Check sheet for the modelled part. Datum: model origin and axes. Units: mm. A direction names the side the tool comes from. Give positions to 0.01 mm unless a question says otherwise; leave off trailing zeros. Use CSV: the item, a comma, the result in double quotes.
from build123d import *

# Parameters (mm, degrees)
SKETCH_1_W             = 23.5
SKETCH_1_H             = 12
EXTRUDE_1_DEPTH        = 650.5
HOLE_WIZARD_M6_1_D     = 5
HOLE_WIZARD_M6_1_DEPTH = 19
HOLE_WIZARD_M6_1_TIP   = 1.502151548
HOLE_WIZARD_M4_1_D     = 3.3
HOLE_WIZARD_M4_1_DEPTH = 15.5
HOLE_WIZARD_M4_1_TIP   = 0.991420021
HOLE_WIZARD_M6_2_D     = 5
HOLE_WIZARD_M6_2_DEPTH = 17
HOLE_WIZARD_M6_2_TIP   = 1.502151548
HOLE_WIZARD_M4_2_D     = 3.3
HOLE_WIZARD_M4_2_DEPTH = 11.5
HOLE_WIZARD_M4_2_TIP   = 0.991420021


with BuildPart() as part:
    # 草图1 → 凸台-拉伸1 (new, symmetric)
    with BuildSketch(Plane(origin=(0, 0, 0), x_dir=(0, 0, -1), z_dir=(1, 0, 0))):
        Polygon((-15, 15), (-11.5, 15), (-11.5, 13.5), (-11, 13.5), (-11, 12), (-9.5, 12), (-9.5, 15), (-8, 15), (-8, 12.5), (-5, 12.5), (-5, 15), (5, 15), (5, 12.5), (8, 12.5), (8, 15), (9.5, 15), (9.5, 12), (11, 12), (11, 13.5), (11.5, 13.5), (11.5, 15), (15, 15), (15, 8), (12.5, 8), (12.5, 5), (15, 5), (15, -5), (12.5, -5), (12.5, -8), (15, -8), (15, -15), (11.5, -15), (11.5, -13.5), (11, -13.5), (11, -12), (9.5, -12), (9.5, -15), (8, -15), (8, -12.5), (5, -12.5), (5, -15), (-5, -15), (-5, -12.5), (-8, -12.5), (-8, -15), (-9.5, -15), (-9.5, -12), (-11, -12), (-11, -13.5), (-11.5, -13.5), (-11.5, -15), (-15, -15), align=None)
        with BuildLine():
            Line((12, -10.5), (12, -8.5))
            ThreePointArc((12, -8.5), (11.853553391, -8.146446609), (11.5, -8))
            Line((11.5, -8), (-11.5, -8))
            ThreePointArc((-11.5, -8), (-11.853553391, -8.146446609), (-12, -8.5))
            Line((-12, -8.5), (-12, -10.5))
            ThreePointArc((-12, -10.5), (-11.853553391, -10.853553391), (-11.5, -11))
            Line((-11.5, -11), (11.5, -11))
            ThreePointArc((11.5, -11), (11.853553391, -10.853553391), (12, -10.5))
        make_face(mode=Mode.SUBTRACT)
        with BuildLine():
            Line((-11.5, 11), (11.5, 11))
            ThreePointArc((11.5, 11), (11.853553391, 10.853553391), (12, 10.5))
            Line((12, 10.5), (12, 8.5))
            ThreePointArc((12, 8.5), (11.853553391, 8.146446609), (11.5, 8))
            Line((11.5, 8), (-11.5, 8))
            ThreePointArc((-11.5, 8), (-11.853553391, 8.146446609), (-12, 8.5))
            Line((-12, 8.5), (-12, 10.5))
            ThreePointArc((-12, 10.5), (-11.853553391, 10.853553391), (-11.5, 11))
        make_face(mode=Mode.SUBTRACT)
        Rectangle(SKETCH_1_W, SKETCH_1_H, mode=Mode.SUBTRACT)
    extrude(amount=EXTRUDE_1_DEPTH, both=True)

    # M6 螺纹孔1
    with Locations(Plane(origin=(0, 0, -15), x_dir=(-1, 0, 0), z_dir=(0, 0, -1))):
        with Locations((-630.5, 0), (-615.5, 0), (342.5, 0), (327.5, 0), (427.5, 0), (412.5, 0), (630.5, 0), (615.5, 0)):
            Hole(HOLE_WIZARD_M6_1_D / 2, depth=HOLE_WIZARD_M6_1_DEPTH)
            with Locations((0, 0, -(HOLE_WIZARD_M6_1_DEPTH + HOLE_WIZARD_M6_1_TIP / 2))):  # 118° drill point
                Cone(0, HOLE_WIZARD_M6_1_D / 2, HOLE_WIZARD_M6_1_TIP, mode=Mode.SUBTRACT)

    # M4 螺纹孔1
    with Locations(Plane.XY.offset(15)):
        with Locations((-460, 0), (-230, 0), (0, 0), (230, 0), (460, 0)):
            Hole(HOLE_WIZARD_M4_1_D / 2, depth=HOLE_WIZARD_M4_1_DEPTH)
            with Locations((0, 0, -(HOLE_WIZARD_M4_1_DEPTH + HOLE_WIZARD_M4_1_TIP / 2))):  # 118° drill point
                Cone(0, HOLE_WIZARD_M4_1_D / 2, HOLE_WIZARD_M4_1_TIP, mode=Mode.SUBTRACT)

    # M6 螺纹孔2
    with Locations(Plane(origin=(0, -15, 0), x_dir=(-1, 0, 0), z_dir=(0, -1, 0))):
        with Locations((310.5, 0), (285.5, 0), (-285.5, 0), (-310.5, 0), (590.5, 0), (470.5, 0)):
            Hole(HOLE_WIZARD_M6_2_D / 2, depth=HOLE_WIZARD_M6_2_DEPTH)
            with Locations((0, 0, -(HOLE_WIZARD_M6_2_DEPTH + HOLE_WIZARD_M6_2_TIP / 2))):  # 118° drill point
                Cone(0, HOLE_WIZARD_M6_2_D / 2, HOLE_WIZARD_M6_2_TIP, mode=Mode.SUBTRACT)

    # M4 螺纹孔2
    with Locations(Plane(origin=(0, -15, 0), x_dir=(-1, 0, 0), z_dir=(0, -1, 0))):
        with Locations((642.5, 0), (615.5, 0)):
            Hole(HOLE_WIZARD_M4_2_D / 2, depth=HOLE_WIZARD_M4_2_DEPTH)
            with Locations((0, 0, -(HOLE_WIZARD_M4_2_DEPTH + HOLE_WIZARD_M4_2_TIP / 2))):  # 118° drill point
                Cone(0, HOLE_WIZARD_M4_2_D / 2, HOLE_WIZARD_M4_2_TIP, mode=Mode.SUBTRACT)


solid = part.part
1. Scan lines: line 1 along Y through (x, z) = (188, 7); line 2 along Y through (x, z) = (225.5, -3); line 3 along Z through (x, y) = (-497, -13.25). Record each from-to range of solid material in increasing order.
Completed:
line 1,"y = -12.5 to -11, -8 to -6, 6 to 8, 11 to 12.5"
line 2,"y = -15 to -11, -8 to -6, 6 to 8, 11 to 15"
line 3,"z = -15 to -11, -9.5 to -8, -5 to 5, 8 to 9.5, 11 to 15"
2. Go/stop test with flat-tipped pins: pin 1 Ø2 at (x, z) = (-615.5, 0) entering from -Y; pin 2 Ø5 at (y, z) = (1.5, 6.5) entering from +X. Record where each tip stops, or that it passes through.
Completed:
pin 1,"stops at y = 6"
pin 2,"passes through"
3. Set-up check for faces 4 (the face through (9, -6, 0)), 5 (the face through (-650.5, 7, 0)): record each of +Z, -Z, +X, -X, +Y, -Y from which the full face is reachable in a straight line by a thin tool's end or side.
Completed:
face 4,"+X, -X"
face 5,"+Z, -Z, -X, +Y, -Y"
4. Sectioned sample at A-A, the plane x = 20. State how many separate pieces and enclosed holes the cut face has, and give its area (3 significant figures).
Completed:
separate pieces,"1"
enclosed holes,"3"
area,"408 mm²"
5. Release check for a two-part mould opening along Z. For faces 1 (the face through (9, 6, 0)), 2 (the face through (9, 0, 15)), 3 (the face through (650.5, 7, 0)) record: released by +Z, released by -Z, zero draft, split by the parting line, or undercut.
Completed:
face 1,"undercut"
face 2,"released by +Z"
face 3,"zero draft"
